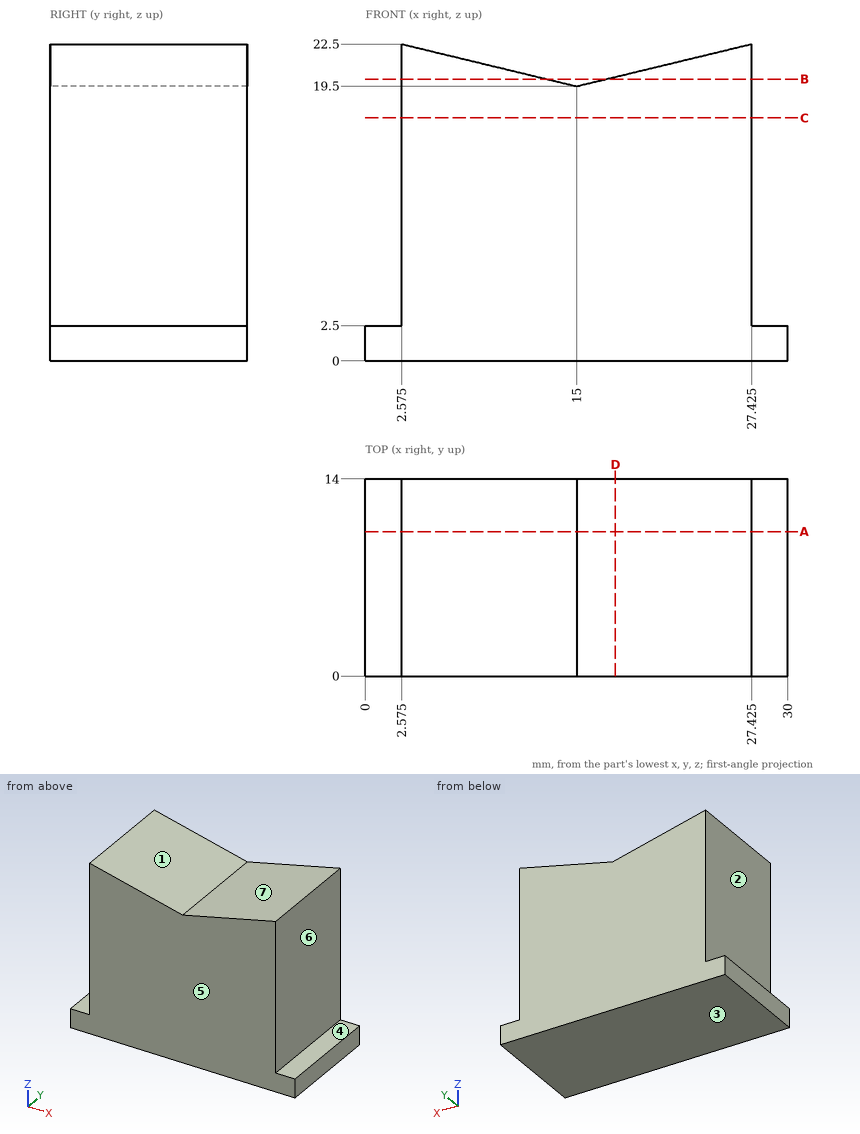
Source: three-view drawing plus pictorial views. Frame: mm from the lowest corner of the part. A direction names the side the tool comes from. Coordinates: 2 decimals unless noted, no trailing zeros. Write each loop counter-clockwise with the first axis right and the second up, starting at its lowest first coordinate (ties: lowest second). Pieces come first, ordered by that corner, then holes. Notation, with made-up numbers: (-35, 78.25) -> (-28, 78.25) arc R26 cw to (-28, 116.25) -> close; hole circle Ø10 at (29, -24). An arc over 180 degrees is marked (long way). Answer as a JSON object with one key per item and string values.
1. Material intervals for line 1 (X direction, y = 7, z = 6.5) (3 decimals); line 2 (Z direction, x = 1.5, y = 2.25); line 3 (Z direction, x = 19.75, y = 10.5), sorted ascending. Write a range as from..to.
Result set:
{"line 1": "x = 2.575..27.425", "line 2": "z = 0..2.5", "line 3": "z = 0..20.65"}
2. Access query for the marked faces 1, 2, 3 and 4. Directions: +Z, -Z, +X, -X, +Y, -Y. A direction counts if a zero-diameter tool reaches every point of the face in a straight line with its end or side. Return the directions, or none.
Result set:
{"face 1": "+Z, +Y, -Y", "face 2": "+Z, -X, +Y, -Y", "face 3": "-Z, +X, -X, +Y, -Y", "face 4": "+Z, +X, +Y, -Y"}
3. Mould query, pull axis X, two halves, no side actions, for the marked faces 5, 6 and 7. Classes: released by +X, released by -X, zero draft, split by the parting line, or undercut.
Result set:
{"face 5": "zero draft", "face 6": "released by +X", "face 7": "undercut"}
4. Section D-D on x = 17.75. Return the cut outline in (y, z).
Result set:
{"outline": "(0, 0) -> (14, 0) -> (14, 20.16) -> (0, 20.16) -> close"}
5. Section B-B on z = 20. Return the cut outline in (x, y) (3 decimals).
Result set:
{"outline": "(2.575, 0) -> (12.929, 0) -> (12.929, 14) -> (2.575, 14) -> close; (17.071, 0) -> (27.425, 0) -> (27.425, 14) -> (17.071, 14) -> close"}
6. Section A-A on y = 10.25. Return the cut outline in (x, z) (3 decimals).
Result set:
{"outline": "(0, 0) -> (30, 0) -> (30, 2.5) -> (27.425, 2.5) -> (27.425, 22.5) -> (15, 19.5) -> (2.575, 22.5) -> (2.575, 2.5) -> (0, 2.5) -> close"}
7. First-contact query: P1, Ø8, axis at y = 6.5, z = 8.5, coming from the +X side (3 decimals); P2, Ø5, axis at x = 16, y = 1.5, coming from the +Z side; P3, Ø6, axis at x = 21, y = 6, coming from the +Z side. Flat tips, straight axial feed; report the tip coordinate or a pass-through.
Result set:
{"P1": "stops at x = 27.425", "P2": "stops at z = 20.35", "P3": "stops at z = 21.67"}
8. Section C-C on z = 17.25. Return the cut outline in (x, y) (3 decimals).
Result set:
{"outline": "(2.575, 0) -> (27.425, 0) -> (27.425, 14) -> (2.575, 14) -> close"}
